Read the model definition and answer for the solid it produces. Units are mm, in the model's axes. Face numbers are marked on the shaded views. A direction names the side the tool comes from. Coordinates: 2 decimals unless noted, no trailing zeros. Loops run counter-clockwise (first coordinate to the right, second up) from the corner with the lowest first, then second, coordinate; pieces in that order, holes last. Notation, with made-up numbers: (24.25, 57) -> (37.25, 57) arc R18 cw to (37.25, 89) -> close; hole circle Ø5 at (37, -35.5). An arc over 180 degrees is marked (long way). Answer as a JSON object with one key per item and string values. Group by question number.
1) Section A-A, the plane x = -7 is taken. Give the vertices of the cut face in (y, z), plus the area to 3 significant figures.
2) Determine the mould class of the marked faces 1, 2, 3 and 4 for opening direction Y: released by +Y, released by -Y, zero draft, split by the parting line, or undercut.
3) Section D-D, the plane x = -1 is taken. Give the vertices of the cut face in (y, z).
4) Flat-ended cylindrical pins translate along their axes: P1, Ø0.5, axis at y = 0.5, z = -0.5, coming from the +X side; P2, Ø0.6, axis at x = 7, z = -5.5, coming from the +Y side; P3, Ø1.6, axis at x = 6.5, z = -5, coming from the -Y side; P4, Ø2.5, axis at x = -7, y = 4.5, coming from the +Z side. Find the tip coordinate at first contact, or state that the pin passes through.
5) Section C-C, the plane z = 1.25 is taken. Give the vertices of the cut face in (x, y).
6) Consider probe 1 along Y at (x, z) = (-7, 0.6); probe 2 along X at (y, z) = (-4.5, 0.6); probe 3 along Z at (x, y) = (-1.5, 1.75). Determine where each line is inside the solid, lowest interval first. Write a range as [from, to].
7) Which of the six approach directions +Z, -Z, +X, -X, +Y, -Y give full straight-line access (tool end or side, diameter ignored) to the marked faces 5, 6, 7 and 8?
8) Section B-B, the plane y = 4.5 is taken. Give the vertices of the cut face in (x, z), plus the area to 3 significant figures.
from build123d import *

# Parameters (mm, degrees)
ESQUISSE1_W             = 18
ESQUISSE1_H             = 13
BOSS_EXTRU_1_DEPTH      = 1.5
ENL_V_MAT_EXTRU_1_REACH = 13.203
ESQUISSE2_R             = 1.5
ESQUISSE3_W             = 2
ESQUISSE3_H             = 12
BOSS_EXTRU_2_DEPTH      = 8
ESQUISSE4_W             = 3
ESQUISSE4_H             = 3
BOSS_EXTRU_3_DEPTH      = 1


with BuildPart() as part:
    # Esquisse1 → Boss.-Extru.1 (new body)
    with BuildSketch(Plane.XY):
        Rectangle(ESQUISSE1_W, ESQUISSE1_H)
    extrude(amount=BOSS_EXTRU_1_DEPTH)

    # Esquisse2 → Enlèv. mat.-Extru.1 (cut, up to next)
    with BuildSketch(Plane(origin=(0, 0, 0), x_dir=(-1, 0, 0), z_dir=(0, 0, -1)), mode=Mode.PRIVATE) as enl_v_mat_extru_1_sk1:
        with Locations((7, 4.5)):
            Circle(ESQUISSE2_R)
    enl_v_mat_extru_1_tool1 = extrude(enl_v_mat_extru_1_sk1.sketch, amount=-ENL_V_MAT_EXTRU_1_REACH, mode=Mode.PRIVATE) & part.part
    enl_v_mat_extru_1 = enl_v_mat_extru_1_tool1.solids().sort_by_distance((-7, 4.5, 0))[0]
    add(enl_v_mat_extru_1, mode=Mode.SUBTRACT)

    # Symétrie1: Enlèv. mat.-Extru.1 across plane
    add(enl_v_mat_extru_1.mirror(Plane.ZX), mode=Mode.SUBTRACT)

    # Esquisse3 → Boss.-Extru.2 (add)
    with BuildSketch(Plane(origin=(0, 0, 0), x_dir=(-1, 0, 0), z_dir=(0, 0, -1))):
        with Locations((-7, 0)):
            Rectangle(ESQUISSE3_W, ESQUISSE3_H)
    extrude(amount=BOSS_EXTRU_2_DEPTH)

    # Esquisse4 → Boss.-Extru.3 (add)
    with BuildSketch(Plane(origin=(0, 0, 0), x_dir=(-1, 0, 0), z_dir=(0, 0, -1))):
        with Locations((0.5, 0)):
            Rectangle(ESQUISSE4_W, ESQUISSE4_H)
    extrude(amount=BOSS_EXTRU_3_DEPTH)


solid = part.part
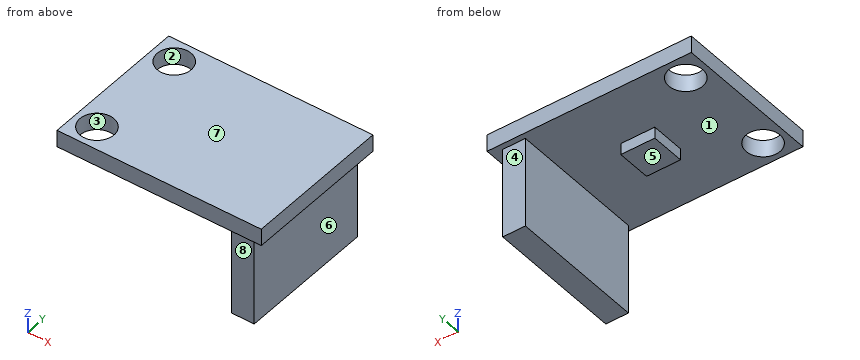
Determined:
{
 "1": {"outline": "(-6.5, 0) -> (-6, 0) -> (-6, 1.5) -> (-6.5, 1.5) -> close; (-3, 0) -> (3, 0) -> (3, 1.5) -> (-3, 1.5) -> close; (6, 0) -> (6.5, 0) -> (6.5, 1.5) -> (6, 1.5) -> close", "area": "10.5 mm²"},
 "2": {"face 1": "zero draft", "face 2": "undercut", "face 3": "undercut", "face 4": "released by +Y"},
 "3": {"outline": "(-6.5, 0) -> (-1.5, 0) -> (-1.5, -1) -> (1.5, -1) -> (1.5, 0) -> (6.5, 0) -> (6.5, 1.5) -> (-6.5, 1.5) -> close"},
 "4": {"P1": "x = 8", "P2": "y = 6", "P3": "y = -6", "P4": "through"},
 "5": {"outline": "(-9, -6.5) -> (9, -6.5) -> (9, 6.5) -> (-9, 6.5) -> close; hole circle Ø3 at (-7, -4.5); hole circle Ø3 at (-7, 4.5)"},
 "6": {"probe 1": "[-6.5, -6], [-3, 3], [6, 6.5]", "probe 2": "[-9, -8.5], [-5.5, 9]", "probe 3": "[0, 1.5]"},
 "7": {"face 5": "-Z, -X, +Y, -Y", "face 6": "-Z, +X, +Y, -Y", "face 7": "+Z, +X, -X, +Y, -Y", "face 8": "-Z, +X, -X, -Y"},
 "8": {"outline": "(-9, 0) -> (-8.5, 0) -> (-8.5, 1.5) -> (-9, 1.5) -> close; (-5.5, 0) -> (6, 0) -> (6, -8) -> (8, -8) -> (8, 0) -> (9, 0) -> (9, 1.5) -> (-5.5, 1.5) -> close", "area": "38.5 mm²"}
}
